from build123d import *

# Parameters (mm, degrees)
F0_R     = 11.2395
F1_DEPTH = 6.35


# Not quite as in the source:
# - ends of sketch curves that miss each other by under 0.0002 mm in the source are joined


with BuildPart() as f1:
    # F0 (on Front) → F1 (new body)
    with BuildSketch(Plane.XZ):
        with BuildLine():
            Line((42.4467651581, 1.27), (33.5675281941, 16.6492895541))
            Line((33.5675281941, 16.6492895541), (19.2425445444, 17.5521669359))
            Line((19.2425445444, 17.5521669359), (7.6766035347, 13.2964561731))
            Line((7.6766035347, 13.2964561731), (5.579663063, 25.4405181745))
            Line((5.579663063, 25.4405181745), (-2.3645964913, 37.3949769354))
            Line((-2.3645964913, 37.3949769354), (-20.1235303163, 37.3949769354))
            ThreePointArc((-20.1235303163, 37.3949769354), (-21.3935303163, 37.054681461), (-22.3232348419, 36.1249769354))
            Line((-22.3232348419, 36.1249769354), (-31.2024718059, 20.7456873813))
            Line((-31.2024718059, 20.7456873813), (-31.1641125036, 20.668391129))
            Line((-31.1641125036, 20.668391129), (-27.8130050023, 13.9157122299))
            Line((-27.8130050023, 13.9157122299), (-24.8577417731, 7.960682843))
            Line((-24.8577417731, 7.960682843), (-24.8218947301, 7.8884489409))
            Line((-24.8218947301, 7.8884489409), (-15.353319828, -3.34766e-05))
            Line((-15.353319828, -3.34766e-05), (-24.8219665561, -7.8881291301))
            Line((-24.8219665561, -7.8881291301), (-24.8578663434, -7.9604670809))
            Line((-24.8578663434, -7.9604670809), (-31.1643564099, -20.6680233587))
            Line((-31.1643564099, -20.6680233587), (-31.2027017544, -20.7452890988))
            Line((-31.2027017544, -20.7452890988), (-22.3232348418, -36.1249769356))
            ThreePointArc((-22.3232348418, -36.1249769356), (-21.9195815404, -36.6510281597), (-21.3935303163, -37.0546814611))
            ThreePointArc((-21.3935303163, -37.0546814611), (-20.7809306909, -37.3084285342), (-20.1235303165, -37.3949769354))
            Line((-20.1235303165, -37.3949769354), (-2.3645964913, -37.3949769354))
            Line((-2.3645964913, -37.3949769354), (-2.3168550697, -37.3231360229))
            Line((-2.3168550697, -37.3231360229), (1.8552556307, -31.0449769354))
            Line((1.8552556307, -31.0449769354), (5.579663063, -25.4405181745))
            Line((5.579663063, -25.4405181745), (7.6765207659, -13.2964418818))
            Line((7.6765207659, -13.2964418818), (19.2425445444, -17.5521669359))
            Line((19.2425445444, -17.5521669359), (25.957862804, -17.1289127727))
            Line((25.957862804, -17.1289127727), (33.5675281941, -16.6492895541))
            Line((33.5675281941, -16.6492895541), (42.4467651581, -1.27))
            ThreePointArc((42.4467651581, -1.27), (42.7870606325, 0), (42.4467651581, 1.27))
        make_face()
        with BuildLine():
            ThreePointArc((-1.8702560234, -22.7067635073), (-22.8434485492, -28.3265135073), (-7.4900060234, -12.9730709815))
            ThreePointArc((-7.4900060234, -12.9730709815), (-3.3760634975, -17.0870135073), (-1.8702560234, -22.7067635073))
        make_face(mode=Mode.SUBTRACT)
        with BuildLine():
            ThreePointArc((-4.7625, -8.248891971), (-4.7625, 8.248891971), (9.525, 0))
            ThreePointArc((9.525, 0), (4.7625, -8.248891971), (-4.7625, -8.248891971))
        make_face(mode=Mode.SUBTRACT)
        with Locations((-13.1097560234, 22.7067635073)):
            Circle(F0_R, mode=Mode.SUBTRACT)
        with Locations((26.2195120463, 0.0001612286)):
            Circle(F0_R, mode=Mode.SUBTRACT)
        with BuildLine():
            Line((43.18, 0), (42.4467651581, 1.27))
            ThreePointArc((42.4467651581, 1.27), (42.7870606325, 0), (42.4467651581, -1.27))
            Line((42.4467651581, -1.27), (43.18, 0))
        make_face()
        with BuildLine():
            ThreePointArc((-22.3232348419, 36.1249769354), (-21.3935303163, 37.054681461), (-20.1235303163, 37.3949769354))
            Line((-20.1235303163, 37.3949769354), (-21.59, 37.3949769354))
            Line((-21.59, 37.3949769354), (-22.3232348419, 36.1249769354))
        make_face()
        with BuildLine():
            Line((-21.59, -37.3949769354), (-20.1235303165, -37.3949769354))
            ThreePointArc((-20.1235303165, -37.3949769354), (-20.7809306909, -37.3084285342), (-21.3935303163, -37.0546814611))
            Line((-21.3935303163, -37.0546814611), (-21.59, -37.3949769354))
        make_face()
        with BuildLine():
            Line((-21.59, -37.3949769354), (-21.3935303163, -37.0546814611))
            ThreePointArc((-21.3935303163, -37.0546814611), (-21.9195815404, -36.6510281597), (-22.3232348418, -36.1249769356))
            Line((-22.3232348418, -36.1249769356), (-21.59, -37.3949769354))
        make_face()
    extrude(amount=F1_DEPTH)


solid = f1.part
The model under review builds one solid part; all positions refer to its coordinate system, in mm. A direction names the side the tool comes from. Round coordinates to 2 decimals unless told otherwise and drop trailing zeros. Loops run counter-clockwise (first coordinate to the right, second up) from the corner with the lowest first, then second, coordinate; pieces in that order, holes last. Notation, with made-up numbers: (-5, -2) - (0, -2) arc R20 ccw to (0, 8) - close; hole circle Ø8 at (70.5, -35). An arc over 180 degrees is marked (long way). Use CSV: the item, a comma, the result in double quotes.
(1) Take a section at C-C, the plane y = -1.5. State how many separate pieces and enclosed holes the cut face has, plus the area to 3 significant figures.
Working result:
separate pieces,"1"
enclosed holes,"4"
area,"1,850 mm^2"
(2) Take a section at A-A, the plane z = 26.5. Give the boundary of the cut face in (x, y).
Working result:
outline,"(-27.88, -6.35) - (-23.69, -6.35) - (-23.69, 0) - (-27.88, 0) - close; (-2.53, -6.35) - (4.88, -6.35) - (4.88, 0) - (-2.53, 0) - close"
(3) The part is to be moulded in two halves that separate along Z. For faces 1 (the flat face through (-20.02, -3.13, -3.89)), 2 (the flat face through (6.613, -3.131, -19.453)), 3 (the flat face through (-20.154, -3.131, 3.999)), 4 (the flat face through (13.541, -3.131, 15.454)), say which applies: pulls with the +Z half, pulls with the -Z half, needs draft (parallel to the pull), parting line crosses it, or undercut.
Working result:
face 1,"undercut"
face 2,"pulls with the -Z half"
face 3,"undercut"
face 4,"pulls with the +Z half"
(4) Machinability: for faces 5 (the flat face through (13.379, -3.131, -15.395)), 6 (the flat face through (26.505, -3.131, 17.094)), 7 (the flat face through (6.643, -3.131, 19.283)), which of the approach directions +Z, -Z, +X, -X, +Y, -Y give a long, thin tool a straight path to every point of the face, cutting with its end or side? Answer none if there is none.
Working result:
face 5,"-Z, +Y, -Y"
face 6,"+Z, +X, +Y, -Y"
face 7,"+Z, +Y, -Y"
(5) Clearance check with flat-ended pins moving along their axes: P1, Ø1.5, axis at x = 24, y = -4.5, coming from the -Z side; P2, Ø2, axis at y = -0.5, z = 1, coming from the -X side. State where each tip first meets the part, or that it passes through.
Working result:
P1,"stops at z = -17.3"
P2,"stops at x = -17.75"
(6) For line 1 (X direction, y = -3.5, z = -5); line 2 (X direction, y = -3, z = 8); line 3 (Z direction, x = 30, y = -1), list the stretches that pass through material, from the lowest coordinate up.
Working result:
line 1,"x = -21.36 to -8.11, 8.11 to 16.15, 36.29 to 40.29"
line 2,"x = -24.88 to -5.17, 5.17 to 18.32, 34.11 to 38.56"
line 3,"z = -16.87 to -10.58, 10.58 to 16.87"
(7) Take a section at B-B, the plane x = 0. Give the boundary of the cut face in (y, z) (3 decimals).
Working result:
outline,"(-6.35, -33.837) - (0, -33.837) - (0, -9.525) - (-6.35, -9.525) - close; (-6.35, 9.525) - (0, 9.525) - (0, 33.837) - (-6.35, 33.837) - close"
